Part model, mm, in its own coordinate system. Face numbers are marked on the shaded views. A direction names the side the tool comes from. Coordinates: 2 decimals unless noted, no trailing zeros. Write each loop counter-clockwise with the first axis right and the second up, starting at its lowest first coordinate (ties: lowest second). Pieces come first, ordered by that corner, then holes. Notation, with made-up numbers: (32.5, 22) - (40.5, 22) arc R18 cw to (40.5, 37) - close; hole circle Ø10 at (67, -8.5). An arc over 180 degrees is marked (long way). Write each question's results on one line, items separated by ' | '.
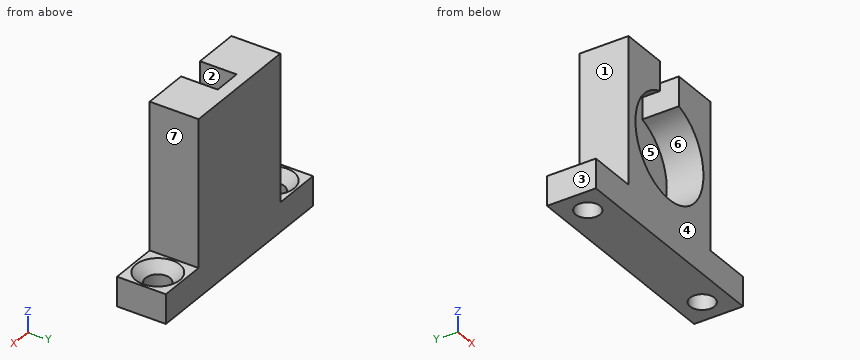
Autodesk Inventor part; units mm, degrees
ref_plane "YZ Plane" through (0, 0, 0) normal (1, 0, 0) x (0, 1, 0)
ref_plane "XZ Plane" through (0, 0, 0) normal (0, 1, 0) x (-1, 0, 0)
ref_plane "XY Plane" through (0, 0, 0) normal (0, 0, 1) x (1, 0, 0)
sketch "Sketch1" plane through (0, 0, 0) normal (0, 0, 1) x (1, 0, 0)
  circle A0 centre (0, 0) radius 1.5875
  circle A1 centre (22.225, 0) radius 1.5875
  line L0 (-3.175, 3.175) -> (25.4, 3.175)
  line L1 (25.4, 3.175) -> (25.4, -3.175)
  line L2 (25.4, -3.175) -> (-3.175, -3.175)
  line L3 (-3.175, -3.175) -> (-3.175, 3.175)
  dimension "d0" = 3.175
  dimension "d1" = 3.175
  dimension "d2" = 22.225
  dimension "d3" = 3.175
  dimension "d4" = 3.175
  dimension "d5" = 3.175
  dimension "d6" = 3.175
extrude "Extrusion1" add sketch "Sketch1" along normal blind 3.81
sketch "Sketch2" plane through (0, 0, 3.81) normal (0, 0, 1) x (1, 0, 0)
  circle A0 centre (22.225, 0) radius 1.5875
  circle A1 centre (0, 0) radius 1.5875
  line L0 (25.4, 3.175) -> (-3.175, 3.175)
  line L1 (-3.175, 3.175) -> (-3.175, -3.175)
  line L2 (-3.175, -3.175) -> (25.4, -3.175)
  line L3 (25.4, -3.175) -> (25.4, 3.175)
  line L4 (3.175, 3.175) -> (19.05, 3.175)
  line L5 (19.05, 3.175) -> (19.05, -3.175)
  line L6 (19.05, -3.175) -> (3.175, -3.175)
  line L7 (3.175, -3.175) -> (3.175, 3.175)
  dimension "d9" = 15.875
  dimension "d10" = 3.175
extrude "Extrusion2" add sketch "Sketch2" along normal blind 19.05 contours L5 L2 L7 L0
sketch "Sketch3" plane through (-3.175, -3.175, 0) normal (0, -1, 0) x (1, 0, 0)
  line L0 (28.575, 0) -> (0, 0)
  line L1 (28.575, 0) -> (28.575, 3.81)
  line L2 (22.225, 3.81) -> (28.575, 3.81)
  line L3 (22.225, 3.81) -> (22.225, 22.86)
  line L4 (6.35, 22.86) -> (22.225, 22.86)
  line L5 (6.35, 3.81) -> (6.35, 22.86)
  line L6 (0, 3.81) -> (6.35, 3.81)
  line L7 (0, 0) -> (0, 3.81)
  line L8 (6.35, 3.81) -> (22.225, 3.81)
  circle A0 centre (14.2875, 12.7) radius 6.604
  line L9 (12.4481, 19.0427) -> (12.4481, 22.86)
  line L10 (16.1269, 19.0427) -> (16.1269, 22.86)
  point P0 (3.175, 0)
  dimension "d13" = 13.208
  dimension "d22" = 12.7
extrude "Extrusion4" cut sketch "Sketch3" against normal blind 4.7625 contours L10 A0 L9 L4 | A0
chamfer "Chamfer1" distance 1.27 angle 45 2 edges at (-1.5875, 0, 3.81) (20.6375, 0, 3.81)
properties part number "potentiometerMountForePlanes" material "ABS Plastic"
(1) Flat gauge pins, fed straight in: P1, Ø4, axis at x = 10, z = 13.5, coming from the -Y side; P2, Ø1.9, axis at y = -2, z = 21, coming from the +X side; P3, Ø1.1, axis at y = -0.5, z = 21.5, coming from the -X side (3 decimals). Where does each tip first touch, or does it go through?
Return value:
P1: stops at y = 1.59 | P2: stops at x = 19.05 | P3: stops at x = 3.175
(2) Two-plate mould, pull along X, no slides. Class the marked faces 4, 5, 6 and 7: released by +X, released by -X, zero draft, split by the parting line, or undercut.
Return value:
face 4: zero draft | face 5: undercut | face 6: undercut | face 7: released by +X
(3) Saw through at C-C on z = 1.5. Write the cut outline in (x, y) (1 decimal).
Return value:
outline: (-3.2, -3.2) - (25.4, -3.2) - (25.4, 3.2) - (-3.2, 3.2) - close; hole circle Ø3.2 at (0, 0); hole circle Ø3.2 at (22.2, 0)
(4) Saw through at B-B on y = 0. Count the separate pieces of the cut face and the enclosed holes in it, then the cut area to 3 significant figures.
Return value:
separate pieces: 3 | enclosed holes: 0 | area: 233 mm^2
(5) 3-axis set-ups, long thin cutter, end or side, ignore diameter. For the marked faces 1, 2 and 3: which of +Z, -Z, +X, -X, +Y, -Y reach the whole face in a straight line?
Return value:
face 1: +Z, -X, +Y, -Y | face 2: +Z, -Y | face 3: +Z, -Z, -X, +Y, -Y
(6) Wall check: line 1 (X direction, y = 0.5, z = 2) (3 decimals); line 2 (Y direction, x = 0, z = 1.7) (1 decimal); line 3 (Z direction, x = 20.25, y = -1). Give the ranges that are in metal, low to high. Write a range as from..to.
Return value:
line 1: x = -3.175..-1.507, 1.507..20.718, 23.732..25.4 | line 2: y = -3.2..-1.6, 1.6..3.2 | line 3: z = 0..3.17
